Study the drawing (mm; zero at the part's minimum x, y, z) and answer. A direction names the side the tool comes from. Round coordinates to 2 decimals unless told otherwise and drop trailing zeros. Order: outer loops, then holes, each group sorted by start corner. A loop starts at its lowest first (then second) coordinate and runs counter-clockwise, first axis right, second up. Notation, with made-up numbers: (41, 38) -> (88, 38) arc R16 cw to (88, 69) -> close; hole circle Ø3 at (13.5, 46). An arc over 180 degrees is marked (long way). Use one line per item in the form item = value.
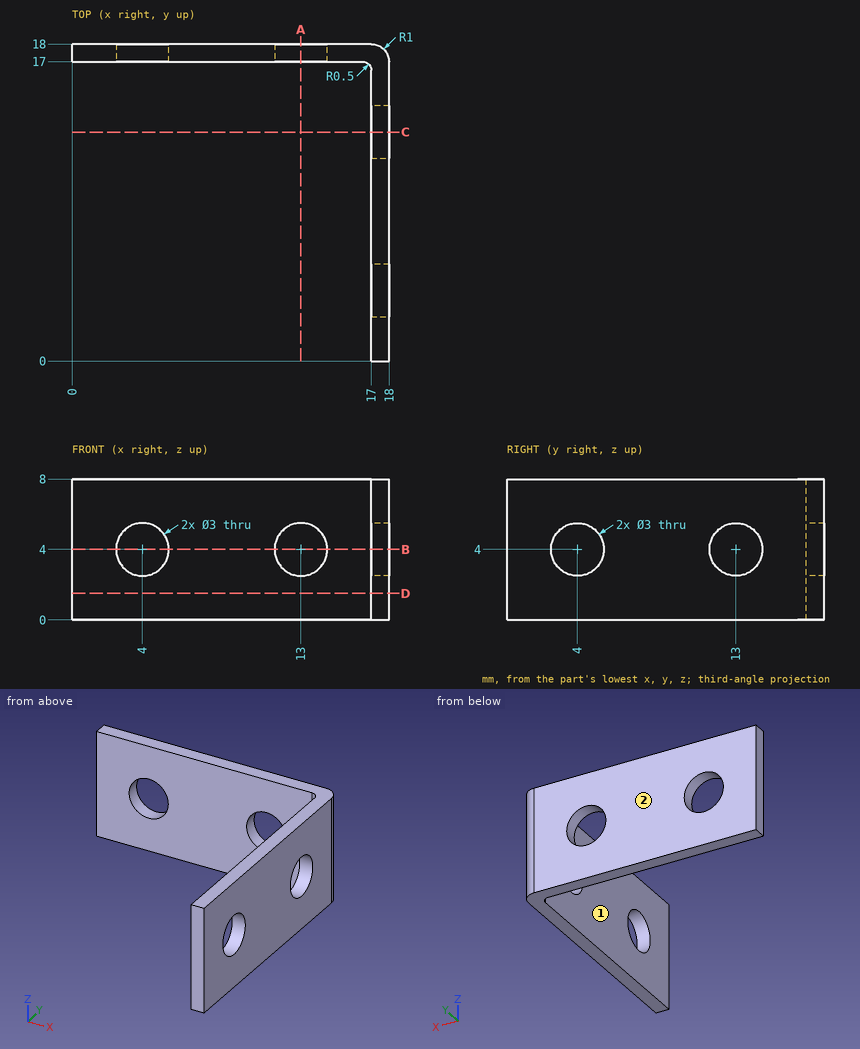
Item 1: The part is cut by section A-A, the plane x = 13. Give the vertices of the cut face in (y, z).
Findings:
outline = (17, 0) -> (18, 0) -> (18, 2.5) -> (17, 2.5) -> close; (17, 5.5) -> (18, 5.5) -> (18, 8) -> (17, 8) -> close
Item 2: The part is cut by section D-D, the plane z = 1.5. Give the vertices of the cut face in (x, y), and give its area (3 significant figures).
Findings:
outline = (0, 17) -> (16.5, 17) arc R0.5 cw to (17, 16.5) -> (17, 0) -> (18, 0) -> (18, 17) arc R1 ccw to (17, 18) -> (0, 18) -> close
area = 34.8 mm^2
Item 3: The part is cut by section B-B, the plane z = 4. Give the vertices of the cut face in (x, y).
Findings:
outline = (0, 17) -> (2.5, 17) -> (2.5, 18) -> (0, 18) -> close; (5.5, 17) -> (11.5, 17) -> (11.5, 18) -> (5.5, 18) -> close; (14.5, 17) -> (16.5, 17) arc R0.5 cw to (17, 16.5) -> (17, 14.5) -> (18, 14.5) -> (18, 17) arc R1 ccw to (17, 18) -> (14.5, 18) -> close; (17, 0) -> (18, 0) -> (18, 2.5) -> (17, 2.5) -> close; (17, 5.5) -> (18, 5.5) -> (18, 11.5) -> (17, 11.5) -> close
Item 4: Consider line 1 along Z through (x, y) = (13, 17.4); line 2 along X through (y, z) = (13.5, 1). Determine where each line is inside the solid, lowest interval first.
Findings:
line_1 = 0 to 2.5, 5.5 to 8
line_2 = 17 to 18
Item 5: Flat-ended cylindrical pins translate along their axes: P1, Ø3, axis at x = 9, z = 3, coming from the -Y side; P2, Ø2.5, axis at y = 11.5, z = 5.5, coming from the -X side; P3, Ø5, axis at x = 12, y = 15.5, coming from the +Z side. Find the tip coordinate at first contact, or state that the pin passes through.
Findings:
P1 = 17
P2 = 17
P3 = 8
Item 6: For the marked faces 1 and 2, determine the directions among +Z, -Z, +X, -X, +Y, -Y from which every point of the face is accessible in a straight line to the end or side of a thin tool.
Findings:
face_1 = +Z, -Z, -X, -Y
face_2 = +Z, -Z, +X, -X, +Y
